Print and shaded views of the part. All mm, measured from the part's lowest x, y and z. A direction names the side the tool comes from. Coordinates: 2 decimals unless noted, no trailing zeros. Order: outer loops, then holes, each group sorted by start corner. A loop starts at its lowest first (then second) coordinate and runs counter-clockwise, first axis right, second up. Notation, with made-up numbers: M 45.25,6 L 79.25,6 A17 cw 79.25,19 Z; hole C 64.5,-3.5 d5. An arc over 180 degrees is marked long. Use a Markdown table: item, result. Add a question column.
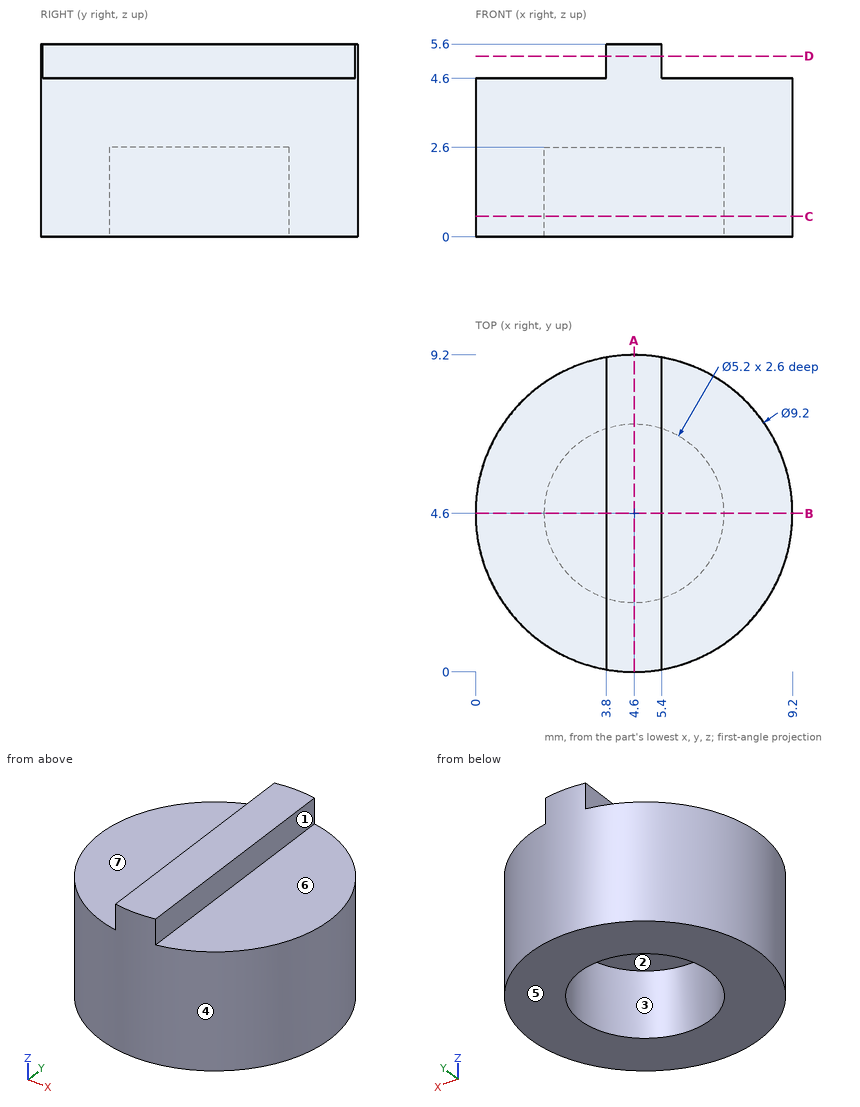
(1) Drill centre lines: line 1 along Z through (x, y) = (5.5, 1.5); line 2 along Y through (x, z) = (4.25, 2.55); line 3 along Z through (x, y) = (3.5, 4.75). Where is each one in solid material? Low to high. Write a range as from..to.
(2) Which spindle directions (+Z, -Z, +X, -X, +Y, -Y) get a long thin tool onto all of the face, cutting with end or side? Do the marked faces 5, 6 and 7. Say none if no direction does.
(3) Slice it at A-A on x = 4.6. Give the cut face in (y, z), and give its area (3 significant figures).
(4) Slice it at C-C on z = 0.6. Give the cut face in (x, y), and give its area (3 significant figures).
(5) Slice it at D-D on z = 5.25. Give the cut face in (x, y).
(6) Drop flat-ended pins along their axis: P1, Ø1, axis at x = 4, y = 2.5, coming from the -Z side; P2, Ø3, axis at x = 7, z = 1, coming from the -Y side; P3, Ø3, axis at y = 2.5, z = 2.5, coming from the -X side; P4, Ø1.5, axis at x = 8, z = 3, coming from the +Y side. Give the stop position or say it passes through.
(7) Slice it at B-B on y = 4.6. Give the cut face in (x, z), and give its area (3 significant figures).
(8) Mould opens along Y. For the marked faces 1, 2, 3 and 4 say: released by +Y, released by -Y, zero draft, split by the parting line, or undercut.
Solutions:
| question | item | result |
|---|---|---|
| 1 | line 1 | 0..4.6 |
| 1 | line 2 | 0.01..2.02, 7.18..9.19 |
| 1 | line 3 | 2.6..4.6 |
| 2 | face 5 | -Z, +X, -X, +Y, -Y |
| 2 | face 6 | +Z, +X, +Y, -Y |
| 2 | face 7 | +Z, -X, +Y, -Y |
| 3 | outline | M 0,0 L 2,0 L 2,2.6 L 7.2,2.6 L 7.2,0 L 9.2,0 L 9.2,5.6 L 0,5.6 Z |
| 3 | area | 38.0 mm² |
| 4 | outline | C 4.6,4.6 d9.2; hole C 4.6,4.6 d5.2 |
| 4 | area | 45.2 mm² |
| 5 | outline | M 3.8,0.07 A4.6 ccw 5.4,0.07 L 5.4,9.13 A4.6 ccw 3.8,9.13 Z |
| 6 | P1 | z = 0 |
| 6 | P2 | y = 0.09 |
| 6 | P3 | x = 0.04 |
| 6 | P4 | y = 8.36 |
| 7 | outline | M 0,0 L 2,0 L 2,2.6 L 7.2,2.6 L 7.2,0 L 9.2,0 L 9.2,4.6 L 5.4,4.6 L 5.4,5.6 L 3.8,5.6 L 3.8,4.6 L 0,4.6 Z |
| 7 | area | 30.4 mm² |
| 8 | face 1 | zero draft |
| 8 | face 2 | undercut |
| 8 | face 3 | undercut |
| 8 | face 4 | split by the parting line |
